```python
from build123d import *

# Parameters (mm, degrees)
ZKOSEN_1_SIZE            = 5
ZKOSEN_2_SIZE            = 5
SKICA3_W                 = 8
SKICA3_H                 = 8
ODEBRAT_VYSUNUT_M1_DEPTH = 66


with BuildPart() as part:
    # Skica1 → Rotovat1 (revolve)
    with BuildSketch(Plane(origin=(0, 0, 0), x_dir=(0, 0, -1), z_dir=(1, 0, 0))):
        Polygon((0, 18), (0, 27.5), (34.5, 27.5), (34.5, 32.5), (65, 32.5), (65, 18), align=None)
    revolve(axis=Axis((0, 0, 25.517724518), (0, 0, -1)))

    # Zkosení1
    zkosen_1_edges = [part.edges().sort_by_distance(p)[0] for p in [
        (0, -27.5, 0),
    ]]
    chamfer(zkosen_1_edges, length=ZKOSEN_1_SIZE)

    # Zkosení2
    zkosen_2_edges = [part.edges().sort_by_distance(p)[0] for p in [
        (0, -32.5, -65),
    ]]
    chamfer(zkosen_2_edges, length=ZKOSEN_2_SIZE)

    # Skica3 → Odebrat vysunutím1 (cut, through all)
    with BuildSketch(Plane.XY):
        with Locations((18, 0)):
            Rectangle(SKICA3_W, SKICA3_H)
    extrude(amount=-ODEBRAT_VYSUNUT_M1_DEPTH, mode=Mode.SUBTRACT)


solid = part.part
```
Can you work these out from the model? Positions are in its coordinate system, mm. A direction names the side the tool comes from. Coordinates: 2 decimals unless noted, no trailing zeros. Write each loop counter-clockwise with the first axis right and the second up, starting at its lowest first coordinate (ties: lowest second). Pieces come first, ordered by that corner, then holes. Notation, with made-up numbers: (46.5, -37) - (98.5, -37) arc R13 ccw to (98.5, -19) - close; hole circle Ø1 at (87.5, 46.25). An arc over 180 degrees is marked (long way). Return JSON: item names as keys, results as strings.
Q1. If we section it at B-B (x = 0): Please give me the cut outline in (y, z).
Computed values:
{"outline": "(-32.5, -60) - (-27.5, -65) - (-18, -65) - (-18, 0) - (-22.5, 0) - (-27.5, -5) - (-27.5, -34.5) - (-32.5, -34.5) - close; (18, -65) - (27.5, -65) - (32.5, -60) - (32.5, -34.5) - (27.5, -34.5) - (27.5, -5) - (22.5, 0) - (18, 0) - close"}
Q2. Please list where these lines run through material, in increasing order: L1, parallel to X at y = 0.5, z = -26.5; L2, parallel to Y at x = 4.5, z = -50.5; L3, parallel to Y at x = -6, z = -47. Write a range as from..to.
Computed values:
{"L1": "x = -27.5..-17.99, 22..27.5", "L2": "y = -32.19..-17.43, 17.43..32.19", "L3": "y = -31.94..-16.97, 16.97..31.94"}
Q3. On a 3-axis mill with a long thin cutter (end or side, diameter ignored), from which of +Z, -Z, +X, -X, +Y, -Y can I reach the whole of each face in a straight line? I mean faces 4 (the flat face through (-18, 6, -65)), 5 (the flat face through (20, 4, -32)), 6 (the flat face through (7, 27, -34.5)). Say none if no direction works.
Computed values:
{"face 4": "-Z, +X, -X, +Y, -Y", "face 5": "+Z, -Z", "face 6": "+Z"}
Q4. Thinking about a two-plate mould opening in X: for faces 1 (the conical face through (-27.15, -6.03, -64.69)), 2 (the flat face through (22, 0, -32)), 3 (the flat face through (-18.2, 0.1, 0)), which applies, +X half, -X half, draft (parallel to the pull), parting line (faces both ways), or undercut?
Computed values:
{"face 1": "parting line", "face 2": "undercut", "face 3": "draft"}
Q5. If we section it at D-D (z = -38.5): Please give me the cut outline in (x, y).
Computed values:
{"outline": "circle Ø65 at (0, 0); hole (17.55, -4) - (22, -4) - (22, 4) - (17.55, 4) arc R18 ccw (long way) to start"}
Q6. If we section it at A-A (y = 0): Please give me the cut outline in (x, z), then the cut area to 3 significant figures.
Computed values:
{"outline": "(-32.5, -60) - (-27.5, -65) - (-18, -65) - (-18, 0) - (-22.5, 0) - (-27.5, -5) - (-27.5, -34.5) - (-32.5, -34.5) - close; (22, -65) - (27.5, -65) - (32.5, -60) - (32.5, -34.5) - (27.5, -34.5) - (27.5, -5) - (22.5, 0) - (22, 0) - close", "area": "1,230 mm2"}
Q7. If we section it at C-C (z = -23): Please give me the cut outline in (x, y).
Computed values:
{"outline": "circle Ø55 at (0, 0); hole (17.55, -4) - (22, -4) - (22, 4) - (17.55, 4) arc R18 ccw (long way) to start"}
Q8. I'm going to push flat-ended pins straight in: pin 1 Ø2 at (x, y) = (-24, -9.5) entering from +Z; pin 2 Ø1 at (y, z) = (10, -58) entering from -X; pin 3 Ø8 at (y, z) = (24.5, -45) entering from +X; pin 4 Ø21.5 at (x, y) = (0, 0) entering from -Z. Where does each tip first touch, or does it pass through?
Computed values:
{"pin 1": "stops at z = -2.31", "pin 2": "stops at x = -31.08", "pin 3": "stops at x = 25.22", "pin 4": "passes through"}
